Here's how the part is built. I have some questions about the finished solid (model axes, mm). A direction names the side the tool comes from. Give positions to 0.01 mm unless a question says otherwise; leave off trailing zeros. Order: outer loops, then holes, each group sorted by start corner. A loop starts at its lowest first (then second) coordinate and runs counter-clockwise, first axis right, second up. Notation, with made-up numbers: M 16,-16.5 L 63,-16.5 A29 ccw 63,3.5 Z; hole C 37,30.25 d5. An arc over 180 degrees is marked long. Use one line per item in the form item = value.
from build123d import *

# Parameters (mm, degrees)
F2_SIZE2 = 0.79375
F2_SIZE  = 0.79375
F5_DEPTH = 2.2352
F6_DEPTH = 25.4


with BuildPart() as f1:
    # F0 (on Right) → F1 (revolve)
    with BuildSketch(Plane.YZ):
        with BuildLine():
            Line((3.3734375, 38.3667), (3.3734375, -1.2065))
            Line((3.3734375, -1.2065), (5.6896, -1.2065))
            Line((5.6896, -1.2065), (5.6896, 0.3175))
            ThreePointArc((5.6896, 0.3175), (5.9499820715, 0.9461179285), (6.5786, 1.2065))
            Line((6.5786, 1.2065), (7.651716578, 1.2065))
            ThreePointArc((7.651716578, 1.2065), (8.3185, 2.3241), (7.651716578, 3.4417))
            Line((7.651716578, 3.4417), (4.9022, 3.4417))
            ThreePointArc((4.9022, 3.4417), (4.4531871939, 3.6276871939), (4.2672, 4.0767))
            Line((4.2672, 4.0767), (4.2672, 38.3667))
            ThreePointArc((4.2672, 38.3667), (3.7087667963, 40.9705920952), (2.1316869154, 43.1165))
            Line((2.1316869154, 43.1165), (1.418192935, 43.1165))
            ThreePointArc((1.418192935, 43.1165), (2.8655068761, 40.9349475226), (3.3734375, 38.3667))
        make_face()
    revolve(axis=Axis((0, 0, 20.955), (0, 0, 1)))

    # F2
    f2_edges = [f1.edges().sort_by_distance(p)[0] for p in [
        (0, -5.6896, -1.2065),
    ]]
    chamfer(f2_edges, length=F2_SIZE, length2=F2_SIZE2)

    # F3 (on face) → F5 (join)
    with BuildSketch(Plane(origin=(0, 0, 1.2065), x_dir=(1, 0, 0), z_dir=(0, 0, -1))):
        with BuildLine():
            ThreePointArc((-7.9248, 3.1851184766), (-7.9607701824, 2.6008906675), (-8.0681373786, 2.0254879633))
            ThreePointArc((-8.0681373786, 2.0254879633), (0, -8.3185), (8.0681373786, 2.0254879633))
            ThreePointArc((8.0681373786, 2.0254879633), (7.9607701824, 2.6008906675), (7.9248, 3.1851184766))
            Line((7.9248, 3.1851184766), (7.9248, 8.1611684277))
            ThreePointArc((7.9248, 8.1611684277), (7.2528781234, 9.2025782422), (6.0271020093, 9.0195855424))
            ThreePointArc((6.0271020093, 9.0195855424), (4.8804481809, 8.1611234409), (3.6136161551, 7.4926110625))
            ThreePointArc((3.6136161551, 7.4926110625), (0, 6.746875), (-3.6136161551, 7.4926110625))
            ThreePointArc((-3.6136161551, 7.4926110625), (-4.8804481809, 8.1611234409), (-6.0271020093, 9.0195855424))
            ThreePointArc((-6.0271020093, 9.0195855424), (-7.2528781234, 9.2025782422), (-7.9248, 8.1611684277))
            Line((-7.9248, 8.1611684277), (-7.9248, 3.1851184766))
        make_face()
        with BuildLine():
            ThreePointArc((3.6136161551, 7.4926110625), (0, 8.3185), (-3.6136161551, 7.4926110625))
            ThreePointArc((-3.6136161551, 7.4926110625), (0, 6.746875), (3.6136161551, 7.4926110625))
        make_face()
    extrude(amount=-F5_DEPTH)

    # F4 (on face) → F6 (cut)
    with BuildSketch(Plane(origin=(0, 0, 1.2065), x_dir=(1, 0, 0), z_dir=(0, 0, -1))):
        with BuildLine():
            ThreePointArc((3.6136161551, 7.4926110625), (0, 8.3185), (-3.6136161551, 7.4926110625))
            ThreePointArc((-3.6136161551, 7.4926110625), (0, 6.746875), (3.6136161551, 7.4926110625))
        make_face()
    extrude(amount=-F6_DEPTH, mode=Mode.SUBTRACT)


solid = f1.part
Q1. I need wall thicknesses on L1, parallel to Y at x = 0, z = 0.45; L2, parallel to X at y = 0, z = 31.5. Which ranges of each line are inside material? Lowest first, please.
Found:
L1 = -5.7 to -3.37, 3.37 to 5.7
L2 = -4.27 to -3.37, 3.37 to 4.27
Q2. I want a section at A-A on z = 5. Write out the boundary of the cut face in (x, y), then the cut area to 3 significant figures.
Found:
outline = C 0,0 d8.53; hole C 0,0 d6.75
area = 21.5 mm²
Q3. On a 3-axis mill with a long thin cutter (end or side, diameter ignored), from which of +Z, -Z, +X, -X, +Y, -Y can I reach the whole of each face in a straight line? I mean faces 4 (the face through (-7.925, -6, 2)), 5 (the face through (0, 0, 3.442)), 6 (the face through (4.166, -0.925, 21.462)), 7 (the face through (7.925, -6, 2)), 8 (the face through (-2, -6.5, 1.206)). Say none if no direction works.
Found:
face_4 = +Z, -Z, -X, -Y
face_5 = none
face_6 = +Z
face_7 = +Z, -Z, +X, -Y
face_8 = -Z
Q4. Thinking about a two-plate mould opening in Z: for faces 1 (the face through (-2.28, -2.486, 20.66)), 2 (the face through (7.962, -2.593, 2.308)), 3 (the face through (-3.33, 1.16, -1.206)), which applies, +Z half, -Z half, draft (parallel to the pull), parting line (faces both ways), or undercut?
Found:
face_1 = undercut
face_2 = draft
face_3 = -Z half
Q5. I'm going to push flat-ended pins straight in: pin 1 Ø4 at (x, z) = (-4, 13.5) entering from +Y; pin 2 Ø5 at (x, z) = (5, 15) entering from -Y; pin 3 Ø8 at (x, z) = (3.5, 23) entering from +Y. Where does each tip first touch, or does it pass through?
Found:
pin_1 = 3.77
pin_2 = -3.46
pin_3 = 4.27
